Here's how the part is built. I have some questions about the finished solid (model axes, mm). A direction names the side the tool comes from. Round coordinates to 2 decimals unless told otherwise and drop trailing zeros. Write each loop counter-clockwise with the first axis right and the second up, starting at its lowest first coordinate (ties: lowest second). Pieces come first, ordered by that corner, then holes. Notation, with made-up numbers: M 29,80.25 L 73,80.25 A11 cw 73,94.25 Z; hole C 68,28.25 d10. An arc over 180 degrees is marked long. Write item = value, one per line. Start each with the question number.
(1) I want a section at A-A (y = -20). List the corners of the cut face in (x, z) for me, and give its area (3 significant figures).
(2) On a 3-axis mill with a long thin cutter (end or side, diameter ignored), from which of +Z, -Z, +X, -X, +Y, -Y can I reach the whole of each face in a straight line? I mean faces 1 (the flat face through (-25.95, 33.02, 0.74)), 2 (the flat face through (-26.84, -26.9, 0.74)), 3 (the cylindrical face through (0, -46, 1)). Say none if no direction works.
(3) I want a section at C-C (x = 15). List the corners of the cut face in (y, z) for me.
(4) Will this pin go through, and if not, where does the flat tip stop? pin 1 Ø2 at (x, y) = (-4.24, -4.24) entering from +Z (3 decimals).
(5) I need wall thicknesses on line 1 along Y through (x, z) = (-27, 0.95); line 2 along X through (y, z) = (-26, 1.3); line 3 along X through (y, z) = (-1.5, 0.3). Which ranges of each line are inside material? Lowest first, please.
```python
from build123d import *

# Parameters (mm, degrees)
SKETCH5_R           = 2.5
SKETCH5_R_2         = 1.25
BOSS_EXTRUDE1_DEPTH = 1.5


with BuildPart() as part:
    # Sketch5 → Boss-Extrude1 (new body)
    with BuildSketch(Plane.XY):
        with BuildLine():
            Line((-34.251979013, 27.180911201), (-31.819805153, 24.748737342))
            ThreePointArc((-31.819805153, 24.748737342), (-30.405591591, 24.162950904), (-28.991378029, 24.748737342))
            Line((-28.991378029, 24.748737342), (-24.748737342, 28.991378029))
            ThreePointArc((-24.748737342, 28.991378029), (-24.162950904, 30.405591591), (-24.748737342, 31.819805153))
            Line((-24.748737342, 31.819805153), (-27.180911201, 34.251979013))
            ThreePointArc((-27.180911201, 34.251979013), (-27.760319437, 35.825792464), (-26.937911168, 37.287383147))
            ThreePointArc((-26.937911168, 37.287383147), (0, 46), (26.937911168, 37.287383147))
            ThreePointArc((26.937911168, 37.287383147), (27.760319437, 35.825792464), (27.180911201, 34.251979013))
            Line((27.180911201, 34.251979013), (24.748737342, 31.819805153))
            ThreePointArc((24.748737342, 31.819805153), (24.162950904, 30.405591591), (24.748737342, 28.991378029))
            Line((24.748737342, 28.991378029), (28.991378029, 24.748737342))
            ThreePointArc((28.991378029, 24.748737342), (30.405591591, 24.162950904), (31.819805153, 24.748737342))
            Line((31.819805153, 24.748737342), (34.251979013, 27.180911201))
            ThreePointArc((34.251979013, 27.180911201), (35.825792464, 27.760319437), (37.287383147, 26.937911168))
            ThreePointArc((37.287383147, 26.937911168), (46, 0), (37.287383147, -26.937911168))
            ThreePointArc((37.287383147, -26.937911168), (35.825792464, -27.760319437), (34.251979013, -27.180911201))
            Line((34.251979013, -27.180911201), (31.819805153, -24.748737342))
            ThreePointArc((31.819805153, -24.748737342), (30.405591591, -24.162950904), (28.991378029, -24.748737342))
            Line((28.991378029, -24.748737342), (24.748737342, -28.991378029))
            ThreePointArc((24.748737342, -28.991378029), (24.162950904, -30.405591591), (24.748737342, -31.819805153))
            Line((24.748737342, -31.819805153), (27.180911201, -34.251979013))
            ThreePointArc((27.180911201, -34.251979013), (27.760319437, -35.825792464), (26.937911168, -37.287383147))
            ThreePointArc((26.937911168, -37.287383147), (0, -46), (-26.937911168, -37.287383147))
            ThreePointArc((-26.937911168, -37.287383147), (-27.760319437, -35.825792464), (-27.180911201, -34.251979013))
            Line((-27.180911201, -34.251979013), (-24.748737342, -31.819805153))
            ThreePointArc((-24.748737342, -31.819805153), (-24.162950904, -30.405591591), (-24.748737342, -28.991378029))
            Line((-24.748737342, -28.991378029), (-28.991378029, -24.748737342))
            ThreePointArc((-28.991378029, -24.748737342), (-30.405591591, -24.162950904), (-31.819805153, -24.748737342))
            Line((-31.819805153, -24.748737342), (-34.251979013, -27.180911201))
            ThreePointArc((-34.251979013, -27.180911201), (-35.825792464, -27.760319437), (-37.287383147, -26.937911168))
            ThreePointArc((-37.287383147, -26.937911168), (-46, 0), (-37.287383147, 26.937911168))
            ThreePointArc((-37.287383147, 26.937911168), (-35.825792464, 27.760319437), (-34.251979013, 27.180911201))
        make_face()
        with Locations((-20, 0)):
            Circle(SKETCH5_R, mode=Mode.SUBTRACT)
        with Locations((-20, 15)):
            Circle(SKETCH5_R_2, mode=Mode.SUBTRACT)
        with Locations((-20, -15)):
            Circle(SKETCH5_R_2, mode=Mode.SUBTRACT)
        with Locations((-15, -20)):
            Circle(SKETCH5_R_2, mode=Mode.SUBTRACT)
        with Locations((0, -20)):
            Circle(SKETCH5_R, mode=Mode.SUBTRACT)
        with Locations((15, -20)):
            Circle(SKETCH5_R_2, mode=Mode.SUBTRACT)
        with Locations((20, -15)):
            Circle(SKETCH5_R_2, mode=Mode.SUBTRACT)
        with Locations((20, 0)):
            Circle(SKETCH5_R, mode=Mode.SUBTRACT)
        with Locations((20, 15)):
            Circle(SKETCH5_R_2, mode=Mode.SUBTRACT)
        with Locations((15, 20)):
            Circle(SKETCH5_R_2, mode=Mode.SUBTRACT)
        with Locations((0, 20)):
            Circle(SKETCH5_R, mode=Mode.SUBTRACT)
        with Locations((-15, 20)):
            Circle(SKETCH5_R_2, mode=Mode.SUBTRACT)
        with Locations((4.242640687, 4.242640687)):
            Circle(SKETCH5_R_2, mode=Mode.SUBTRACT)
        with Locations((-4.242640687, 4.242640687)):
            Circle(SKETCH5_R_2, mode=Mode.SUBTRACT)
        with Locations((-4.242640687, -4.242640687)):
            Circle(SKETCH5_R_2, mode=Mode.SUBTRACT)
        with Locations((4.242640687, -4.242640687)):
            Circle(SKETCH5_R_2, mode=Mode.SUBTRACT)
    extrude(amount=BOSS_EXTRUDE1_DEPTH)


solid = part.part
```
Returned:
q1.outline = M -41.42,0 L -16.25,0 L -16.25,1.5 L -41.42,1.5 Z; M -13.75,0 L -2.5,0 L -2.5,1.5 L -13.75,1.5 Z; M 2.5,0 L 13.75,0 L 13.75,1.5 L 2.5,1.5 Z; M 16.25,0 L 41.42,0 L 41.42,1.5 L 16.25,1.5 Z
q1.area = 109 mm²
q2.face_1 = +Z, -Z, -X
q2.face_2 = +Z, -Z
q2.face_3 = +Z, -Z, -Y
q3.outline = M -43.49,0 L -21.25,0 L -21.25,1.5 L -43.49,1.5 Z; M -18.75,0 L 18.75,0 L 18.75,1.5 L -18.75,1.5 Z; M 21.25,0 L 43.49,0 L 43.49,1.5 L 21.25,1.5 Z
q4.pin_1 = through
q5.line_1 = -37.24 to -34.07, -26.74 to 26.74, 34.07 to 37.24
q5.line_2 = -37.95 to -33.07, -27.74 to 27.74, 33.07 to 37.95
q5.line_3 = -45.98 to -22, -18 to 18, 22 to 45.98
